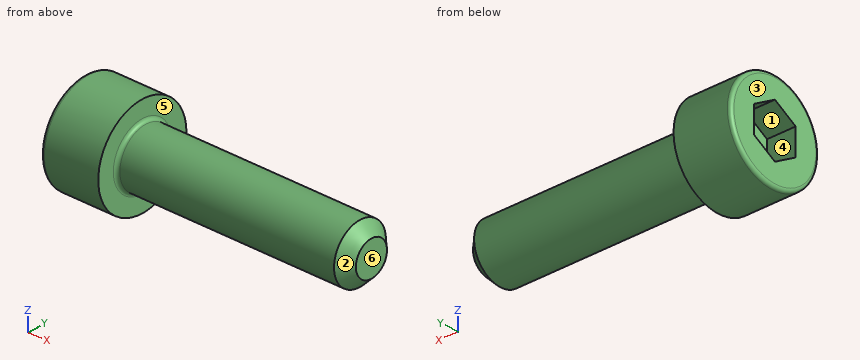
from build123d import *

# Parameters (mm, degrees)
CUT_EXTRUDE_1_DEPTH = 2.5
FILLET_1_R          = 0.3
CHAMFER_1_SIZE      = 1


with BuildPart() as part:
    # Эскиз1 → Повернуть1 (revolve)
    with BuildSketch(Plane.XY):
        Polygon((0, 0), (0, 4.25), (5, 4.25), (5, 2.5), (25, 2.5), (25, 0), align=None)
    revolve(axis=Axis((25, 0, 0), (-1, 0, 0)))

    # Эскиз2 → Вырез-Вытянуть1 (cut)
    with BuildSketch(Plane.ZY):
        Polygon((-1.154700538, 2), (-2.309401077, 0), (-1.154700538, -2), (1.154700538, -2), (2.309401077, 0), (1.154700538, 2), align=None)
    extrude(amount=-CUT_EXTRUDE_1_DEPTH, mode=Mode.SUBTRACT)

    # Скругление1
    fillet_1_edges = [part.edges().sort_by_distance(p)[0] for p in [
        (5, -2.5, 0),
        (0, -4.25, 0),
    ]]
    fillet(fillet_1_edges, radius=FILLET_1_R)

    # Фаска1
    chamfer_1_edges = [part.edges().sort_by_distance(p)[0] for p in [
        (25, -2.5, 0),
    ]]
    chamfer(chamfer_1_edges, length=CHAMFER_1_SIZE)


solid = part.part
CAD build for the part. Positions are in the model's coordinates, mm. Face numbers are marked on the shaded views. A direction names the side the tool comes from. Give positions to 0.01 mm unless a question says otherwise; leave off trailing zeros. Loops run counter-clockwise (first coordinate to the right, second up) from the corner with the lowest first, then second, coordinate; pieces in that order, holes last. Notation, with made-up numbers: M 84,-18 L 118,-18 A25 cw 118,4 Z; hole C 17.5,40.25 d3. An arc over 180 degrees is marked long. Answer in a Markdown table with one row per item. Add a question column.
Item 1: Mould opens along Y. For the marked faces 1, 2 and 3 say: +Y half, -Y half, draft (parallel to the pull), parting line (faces both ways), or undercut.
Item 2: Band-saw the part on A-A on x = 1.75. Give the cut face in (y, z).
Item 3: Drop flat-ended pins along their axis: P1, Ø0.7, axis at x = 1, z = 0.5, coming from the +Y side; P2, Ø2, axis at y = 0.5, z = 0.5, coming from the -X side; P3, Ø1, axis at x = 4, z = -2.5, coming from the +Y side. Give the stop position or say it passes through.
Item 4: Band-saw the part on B-B on z = 0. Give the cut face in (x, y).
Item 5: Tool access for the marked faces 4, 5 and 6: list every direction of +Z, -Z, +X, -X, +Y, -Y with a clear straight run to the whole face (end or side of a thin tool).
Item 6: Probe probe 1 along X at (y, z) = (-0.75, 2.75); probe 2 along Z at (x, y) = (1.75, 1.5); probe 3 along Z at (x, y) = (19.5, 2). List the from-to ranges inside material, lowest first.
Item 7: Band-saw the part on C-C on x = 9. Give the cut face in (y, z).
Reply:
| question | item | result |
|---|---|---|
| 1 | face 1 | undercut |
| 1 | face 2 | parting line |
| 1 | face 3 | draft |
| 2 | outline | C 0,0 d8.5; hole M -2,-1.15 L 0,-2.31 L 2,-1.15 L 2,1.15 L 0,2.31 L -2,1.15 Z |
| 3 | P1 | stops at y = 4.25 |
| 3 | P2 | stops at x = 2.5 |
| 3 | P3 | stops at y = 3.75 |
| 4 | outline | M 0,-3.95 A0.3 ccw 0.3,-4.25 L 5,-4.25 L 5,-2.8 A0.3 cw 5.3,-2.5 L 24,-2.5 L 25,-1.5 L 25,1.5 L 24,2.5 L 5.3,2.5 A0.3 cw 5,2.8 L 5,4.25 L 0.3,4.25 A0.3 ccw 0,3.95 L 0,2 L 2.5,2 L 2.5,-2 L 0,-2 Z |
| 5 | face 4 | -X |
| 5 | face 5 | +X |
| 5 | face 6 | +Z, -Z, +X, +Y, -Y |
| 6 | probe 1 | x = 0 to 5 |
| 6 | probe 2 | z = -3.98 to -1.44, 1.44 to 3.98 |
| 6 | probe 3 | z = -1.5 to 1.5 |
| 7 | outline | C 0,0 d5 |
